Geometry check sheet. Reference: drawing and pictorial views, mm from the part's lowest x, y, z. Give positions to 0.01 mm unless a question says otherwise; leave off trailing zeros. Write each loop counter-clockwise with the first axis right and the second up, starting at its lowest first coordinate (ties: lowest second). Pieces come first, ordered by that corner, then holes. Notation, with made-up numbers: M 39.25,64.25 L 48.25,64.25 A28 cw 48.25,82.25 Z; hole C -2.75,-26 d3. An arc over 180 degrees is marked long. Answer as a JSON object with one key per item and string values.
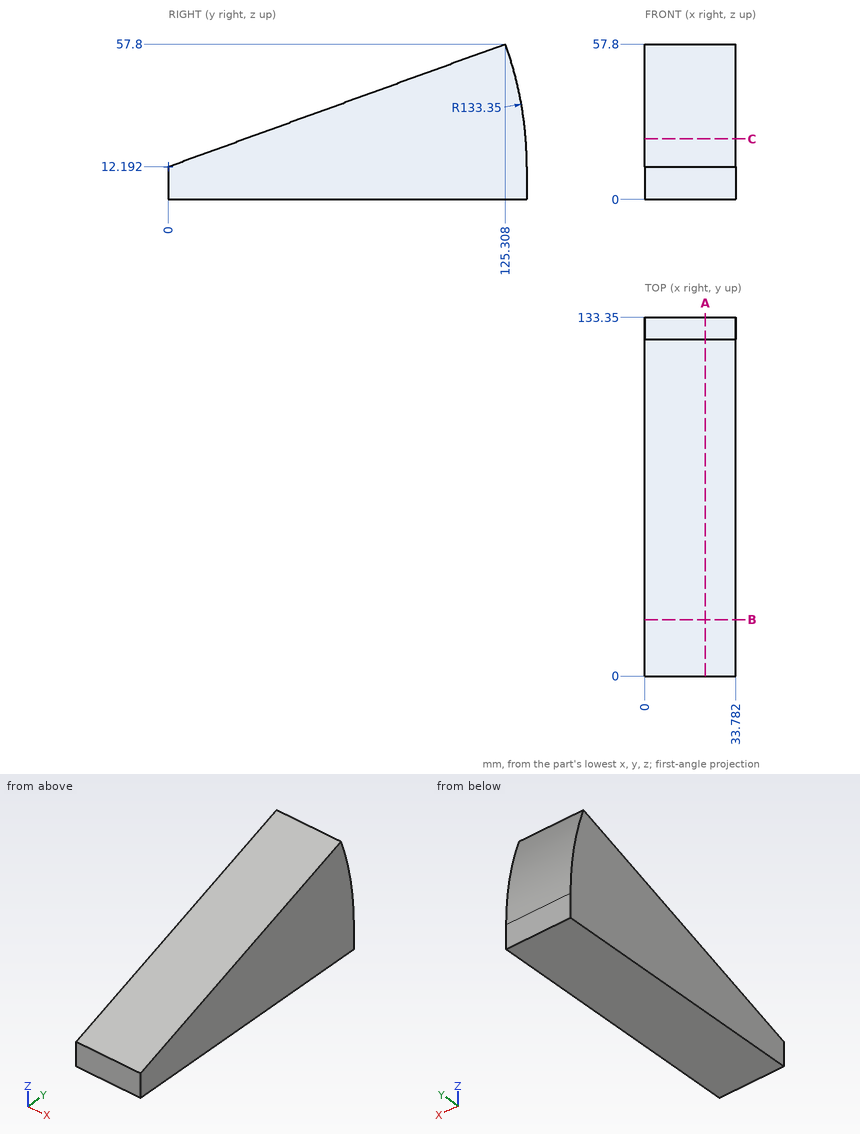
1) Thickness scan on L1, parallel to Z at x = 30, y = 122; L2, parallel to Z at x = 3.5, y = 72.5. Record the ranges inside material, lowest first.
Completed:
{"L1": "z = 0 to 56.6", "L2": "z = 0 to 38.58"}
2) Go/stop test with flat-tipped pins: pin 1 (12 mm diameter, centred on x = 22, z = 33, fed in from +Y) (1 decimal); pin 2 (6 mm diameter, centred on x = 29, y = 36.5, fed in from +Z); pin 3 (10 mm diameter, centred on x = 14, y = 112, fed in from -Z); pin 4 (12 mm diameter, centred on x = 10, y = 76, fed in from +Z). Record where each tip stops, or that it passes through.
Completed:
{"pin 1": "stops at y = 132.5", "pin 2": "stops at z = 26.57", "pin 3": "stops at z = 0", "pin 4": "stops at z = 42.04"}
3) Section check B-B on y = 21. Record the boundary of the cut face in (x, z) (1 decimal).
Completed:
{"outline": "M 0,0 L 33.8,0 L 33.8,19.8 L 0,19.8 Z"}
4) Section check A-A on x = 22.5. Record the boundary of the cut face in (y, z), and give its area (3 significant figures).
Completed:
{"outline": "M 0,0 L 133.35,0 L 133.35,12.19 A133.35 ccw 125.31,57.8 L 0,12.19 Z", "area": "4,730 mm2"}
5) Section check C-C on z = 22.5. Record the boundary of the cut face in (x, y), and give its area (3 significant figures).
Completed:
{"outline": "M 0,28.32 L 33.78,28.32 L 33.78,132.95 L 0,132.95 Z", "area": "3,530 mm2"}
